Source: CAD feature listing. Evaluate the final solid. Frame: model axes, mm. Give positions to 0.01 mm unless a question says otherwise; leave off trailing zeros. Loops run counter-clockwise (first coordinate to the right, second up) from the corner with the lowest first, then second, coordinate; pieces in that order, holes last.
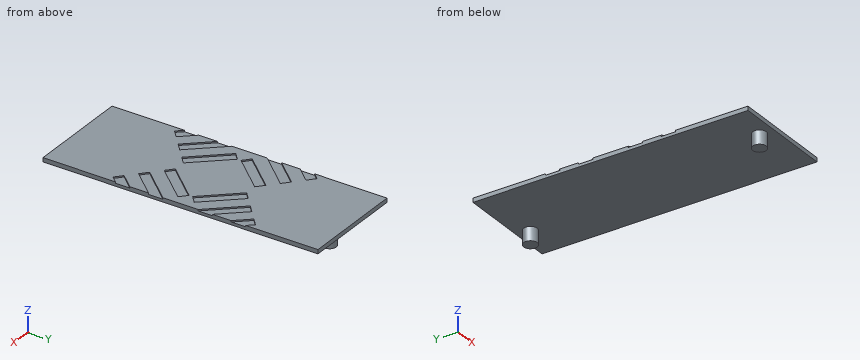
from build123d import *

# Parameters (mm, degrees)
SKETCH1_W           = 225
SKETCH1_H           = 200
BOSS_EXTRUDE1_DEPTH = 3
CUT_EXTRUDE1_DEPTH  = 1
SKETCH4_R           = 4.9
BOSS_EXTRUDE2_DEPTH = 10
SKETCH5_W           = 75
SKETCH5_H           = 200
CUT_EXTRUDE2_DEPTH  = 10


with BuildPart() as part:
    # Sketch1 → Boss-Extrude1 (new body)
    with BuildSketch(Plane.XY):
        with Locations((112.5, 100)):
            Rectangle(SKETCH1_W, SKETCH1_H)
    extrude(amount=BOSS_EXTRUDE1_DEPTH)

    # Sketch2 → Cut-Extrude1 (cut)
    with BuildSketch(Plane.XY.offset(3)):
        Polygon((21.176597363, 159.100101172), (43.100604044, 183.764608689), (48.332469275, 179.114061817), (26.408462593, 154.4495543), align=None)
        Polygon((9.218048264, 169.729922593), (31.142054945, 194.39443011), (36.373920176, 189.743883238), (14.449913495, 165.079375722), align=None)
        Polygon((33.135146462, 148.470279751), (55.059153143, 173.134787267), (60.291018374, 168.484240396), (38.367011692, 143.819732879), align=None)
        Polygon((45.093695561, 137.840458329), (67.017702242, 162.504965846), (72.249567473, 157.854418974), (50.325560791, 133.189911458), align=None)
        Polygon((57.05224466, 127.210636908), (78.976251341, 151.875144425), (84.208116572, 147.224597553), (62.28410989, 122.560090036), align=None)
        Polygon((69.010793758, 116.580815487), (90.93480044, 141.245323003), (96.166665671, 136.594776132), (74.242658989, 111.930268615), align=None)
        Polygon((80.969342857, 105.950994066), (102.893349539, 130.615501582), (108.12521477, 125.96495471), (86.201208088, 101.300447194), align=None)
        Polygon((116.844990154, 74.061529802), (138.768996836, 98.726037318), (144.000862066, 94.075490447), (122.076855385, 69.41098293), align=None)
        Polygon((128.803539253, 63.431708381), (150.727545935, 88.096215897), (155.959411165, 83.445669025), (134.035404484, 58.781161509), align=None)
        Polygon((140.762088352, 52.801886959), (162.686095033, 77.466394476), (167.917960264, 72.815847604), (145.993953583, 48.151340087), align=None)
        Polygon((152.720637451, 42.172065538), (174.644644132, 66.836573055), (179.876509363, 62.186026183), (157.952502682, 37.521518666), align=None)
        Polygon((164.67918655, 31.542244117), (186.603193231, 56.206751633), (191.835058462, 51.556204761), (169.911051781, 26.891697245), align=None)
        Polygon((176.637735649, 20.912422695), (198.56174233, 45.576930212), (203.793607561, 40.92638334), (181.86960088, 16.261875824), align=None)
        Polygon((188.596284748, 10.282601274), (210.520291429, 34.947108791), (215.75215666, 30.296561919), (193.828149979, 5.632054402), align=None)
        Polygon((198.591537407, 154.4495543), (176.667530725, 179.114061817), (181.899395956, 183.764608689), (203.823402637, 159.100101172), align=None)
        Polygon((210.550086505, 165.079375721), (188.626079824, 189.743883238), (193.857945055, 194.39443011), (215.781951736, 169.729922593), align=None)
        Polygon((186.632988308, 143.819732879), (164.708981626, 168.484240395), (169.940846857, 173.134787267), (191.864853538, 148.470279751), align=None)
        Polygon((174.674439209, 133.189911458), (152.750432527, 157.854418974), (157.982297758, 162.504965846), (179.906304439, 137.840458329), align=None)
        Polygon((162.71589011, 122.560090036), (140.791883428, 147.224597553), (146.023748659, 151.875144425), (167.94775534, 127.210636908), align=None)
        Polygon((150.757341011, 111.930268615), (128.833334329, 136.594776132), (134.06519956, 141.245323003), (155.989206242, 116.580815487), align=None)
        Polygon((138.798791912, 101.300447194), (116.87478523, 125.96495471), (122.106650461, 130.615501582), (144.030657143, 105.950994066), align=None)
        Polygon((102.923144615, 69.41098293), (80.999137934, 94.075490447), (86.231003164, 98.726037318), (108.155009846, 74.061529802), align=None)
        Polygon((90.964595516, 58.781161509), (69.040588835, 83.445669025), (74.272454065, 88.096215897), (96.196460747, 63.431708381), align=None)
        Polygon((79.006046417, 48.151340087), (57.082039736, 72.815847604), (62.313904967, 77.466394476), (84.237911648, 52.801886959), align=None)
        Polygon((67.047497318, 37.521518666), (45.123490637, 62.186026183), (50.355355868, 66.836573055), (72.279362549, 42.172065538), align=None)
        Polygon((55.088948219, 26.891697245), (33.164941538, 51.556204761), (38.396806769, 56.206751633), (60.32081345, 31.542244117), align=None)
        Polygon((43.13039912, 16.261875824), (21.206392439, 40.92638334), (26.43825767, 45.576930212), (48.362264351, 20.912422695), align=None)
        Polygon((31.171850021, 5.632054402), (9.24784334, 30.296561919), (14.479708571, 34.947108791), (36.403715252, 10.282601274), align=None)
    extrude(amount=-CUT_EXTRUDE1_DEPTH, mode=Mode.SUBTRACT)

    # Sketch4 → Boss-Extrude2 (add)
    with BuildSketch(Plane(origin=(0, 0, 0), x_dir=(-1, 0, 0), z_dir=(0, 0, -1))):
        with Locations((-102.5, 10)):
            Circle(SKETCH4_R)
        with Locations((-122.5, 190)):
            Circle(SKETCH4_R)
    extrude(amount=BOSS_EXTRUDE2_DEPTH)

    # Sketch5 → Cut-Extrude2 (cut)
    with BuildSketch(Plane(origin=(0, 0, 0), x_dir=(-1, 0, 0), z_dir=(0, 0, -1))):
        with Locations((-37.5, 100)):
            Rectangle(SKETCH5_W, SKETCH5_H)
        with Locations((-187.5, 100)):
            Rectangle(SKETCH5_W, SKETCH5_H)
    extrude(amount=-CUT_EXTRUDE2_DEPTH, mode=Mode.SUBTRACT)


solid = part.part
1) Ray query, probe 1 along Z at (x, y) = (108, 184); probe 2 along Y at (x, z) = (103, -3); probe 3 along Y at (x, z) = (124, -8). Return the intervals inside material, ascending.
Checks:
probe 1: z = 0 to 3
probe 2: y = 5.13 to 14.87
probe 3: y = 185.34 to 194.66
2) Cut plane C-C (x = 114). Return loops of the section in (y, z), and give its area (3 significant figures).
Checks:
outline: (0, 0) - (200, 0) - (200, 3) - (0, 3) - close
area: 600 mm2
3) Cut plane B-B (z = -7.25). Return loops of the section in (x, y).
Checks:
outline: circle Ø9.8 at (102.5, 10); circle Ø9.8 at (122.5, 190)
4) Contact query for flat-ended pins moving along their axis: P1, Ø22.5, axis at x = 121, y = 59, coming from the -Z side; P2, Ø3, axis at x = 78, y = 55, coming from the +Z side; P3, Ø4, axis at x = 141.5, z = -3, coming from the -Y side; P4, Ø6, axis at x = 95.5, z = -6, coming from the +Y side. Output: stop coordinate, or through.
Checks:
P1: stops at z = 0
P2: stops at z = 2
P3: passes through
P4: stops at y = 12.83
5) Cut plane D-D (y = 71.5). Return loops of the section in (x, z), and give its area (3 significant figures).
Checks:
outline: (75, 0) - (150, 0) - (150, 3) - (145.34, 3) - (145.34, 2) - (135.98, 2) - (135.98, 3) - (123.93, 3) - (123.93, 2) - (119.73, 2) - (119.73, 3) - (105.27, 3) - (105.27, 2) - (101.07, 2) - (101.07, 3) - (89.02, 3) - (89.02, 2) - (79.66, 2) - (79.66, 3) - (75, 3) - close
area: 198 mm2
6) Cut plane A-A (y = 10). Return loops of the section in (x, z).
Checks:
outline: (75, 0) - (97.6, 0) - (97.6, -10) - (107.4, -10) - (107.4, 0) - (150, 0) - (150, 3) - (75, 3) - close
